from build123d import *

# Parameters (mm, degrees)
SKETCH1_R                                   = 155.575
SKETCH1_R_2                                 = 7.9375
BOSS_EXTRUDE1_DEPTH                         = 4.7625
FILLET1_R                                   = 12.7
FILLET4_R                                   = 2.54
CSK_FOR_1_4_FLAT_HEAD_MACHINE_SCREW_2_COUNT = 2
CSK_FOR_1_4_FLAT_HEAD_MACHINE_SCREW_2_PITCH = 255.715651102
CSK_FOR_1_4_FLAT_HEAD_MACHINE_SCREW_3_COUNT = 2
CSK_FOR_1_4_FLAT_HEAD_MACHINE_SCREW_3_PITCH = 255.715651102


with BuildPart() as part:
    # Sketch1 → Boss-Extrude1 (new body)
    with BuildSketch(Plane.XY):
        Circle(SKETCH1_R)
        with BuildLine():
            ThreePointArc((-125.107792883, -62.16212802), (-120.983748909, 69.85), (-8.719914422, 139.427590858))
            Line((-8.719914422, 139.427590858), (-12.49892387, 7.216257061))
            Line((-12.49892387, 7.216257061), (-125.107792883, -62.16212802))
        make_face(mode=Mode.SUBTRACT)
        with BuildLine():
            ThreePointArc((8.719914422, 139.427590858), (120.983748909, 69.85), (125.107792883, -62.16212802))
            Line((125.107792883, -62.16212802), (12.49892387, 7.216257061))
            Line((12.49892387, 7.216257061), (8.719914422, 139.427590858))
        make_face(mode=Mode.SUBTRACT)
        with BuildLine():
            ThreePointArc((116.38787846, -77.265462838), (0, -139.7), (-116.38787846, -77.265462838))
            Line((-116.38787846, -77.265462838), (0, -14.432514122))
            Line((0, -14.432514122), (116.38787846, -77.265462838))
        make_face(mode=Mode.SUBTRACT)
        with BuildLine():
            Line((-12.585726429, 4.179407795), (-12.694815268, 0.362857143))
            ThreePointArc((-12.694815268, 0.362857143), (-10.998522628, -6.35), (-6.03316413, -11.17546109))
            Line((-6.03316413, -11.17546109), (-2.673389891, -12.98926271))
            Line((-2.673389891, -12.98926271), (-112.467905529, -72.262730545))
            ThreePointArc((-112.467905529, -72.262730545), (-120.983748909, -69.85), (-118.815313164, -61.268698026))
            Line((-118.815313164, -61.268698026), (-12.585726429, 4.179407795))
        make_face(mode=Mode.SUBTRACT)
        with BuildLine():
            ThreePointArc((118.815313164, -61.268698026), (120.983748909, -69.85), (112.467905529, -72.262730545))
            Line((112.467905529, -72.262730545), (2.673389891, -12.98926271))
            Line((2.673389891, -12.98926271), (6.03316413, -11.17546109))
            ThreePointArc((6.03316413, -11.17546109), (10.998522628, -6.35), (12.694815268, 0.362857143))
            Line((12.694815268, 0.362857143), (12.585726429, 4.179407795))
            Line((12.585726429, 4.179407795), (118.815313164, -61.268698026))
        make_face(mode=Mode.SUBTRACT)
        Circle(SKETCH1_R_2, mode=Mode.SUBTRACT)
        with BuildLine():
            ThreePointArc((-6.347407634, 133.531428571), (0, 139.7), (6.347407634, 133.531428571))
            Line((6.347407634, 133.531428571), (9.938137929, 7.907174875))
            ThreePointArc((9.938137929, 7.907174875), (0, 12.7), (-9.938137929, 7.907174875))
            Line((-9.938137929, 7.907174875), (-6.347407634, 133.531428571))
        make_face(mode=Mode.SUBTRACT)
    extrude(amount=-BOSS_EXTRUDE1_DEPTH)

    # Fillet1
    fillet1_edges = [part.edges().sort_by_distance(p)[0] for p in [
        (12.49892387, 7.216257061, -2.38125),
        (0, -14.432514122, -2.38125),
        (-12.49892387, 7.216257061, -2.38125),
    ]]
    fillet(fillet1_edges, radius=FILLET1_R)

    # Fillet4
    fillet4_edges = [part.edges().sort_by_distance(p)[0] for p in [
        (12.585726429, 4.179407795, -2.38125),
        (2.673389891, -12.98926271, -2.38125),
        (-2.673389891, -12.98926271, -2.38125),
        (-12.585726429, 4.179407795, -2.38125),
        (-9.938137929, 7.907174875, -2.38125),
        (9.938137929, 7.907174875, -2.38125),
    ]]
    fillet(fillet4_edges, radius=FILLET4_R)

    # Sketch4 → CSK for 1/4 Flat Head Machine Screw (100)1 (revolve, cut)
    with BuildSketch(Plane(origin=(0, 147.6375, 0), x_dir=(0, -1, 0), z_dir=(1, 0, 0))):
        Polygon((0, 0), (0, 4.7625), (3.3782, 4.7625), (3.3782, 2.568232241), (6.4389, 0), align=None)
    csk_for_1_4_flat_head_machine_screw_100 = revolve(axis=Axis((0, 147.6375, 6.35), (0, 0, -1)), mode=Mode.SUBTRACT)

    # CSK for 1_4 Flat Head Machine Screw  2: CSK for 1/4 Flat Head Machine Screw (100)1 ×2
    with Locations(*[Vector(0.5, -0.866025404, 0) * (i * CSK_FOR_1_4_FLAT_HEAD_MACHINE_SCREW_2_PITCH) for i in range(1, CSK_FOR_1_4_FLAT_HEAD_MACHINE_SCREW_2_COUNT)]):
        add(csk_for_1_4_flat_head_machine_screw_100, mode=Mode.SUBTRACT)

    # CSK for 1_4 Flat Head Machine Screw  3: CSK for 1/4 Flat Head Machine Screw (100)1 ×2
    with Locations(*[Vector(-0.5, -0.866025404, 0) * (i * CSK_FOR_1_4_FLAT_HEAD_MACHINE_SCREW_3_PITCH) for i in range(1, CSK_FOR_1_4_FLAT_HEAD_MACHINE_SCREW_3_COUNT)]):
        add(csk_for_1_4_flat_head_machine_screw_100, mode=Mode.SUBTRACT)


solid = part.part
The listing builds one solid part. Answer for the finished solid, in the listing's coordinates (mm). A direction names the side the tool comes from. Give positions to 0.01 mm unless a question says otherwise; leave off trailing zeros. Write each loop counter-clockwise with the first axis right and the second up, starting at its lowest first coordinate (ties: lowest second). Pieces come first, ordered by that corner, then holes.
1) Section A-A (x = -57.5) is taken. Write down the section's boundary in (y, z), and give its area (3 significant figures).
2) For a pull along Y with two mould halves and no side action, classify faces 3 (the face through (-130.3, -71.2, -2.4)), 4 (the face through (-1, -11, 0)), 5 (the face through (72.47, -29.73, -2.35)) as pulls with the +Y half, pulls with the -Y half, needs draft (parallel to the pull), parting line crosses it, or undercut.
3) Section B-B (y = -52) is taken. Write down the section's boundary in (x, z).
4) Section C-C (y = 111) is taken. Write down the section's boundary in (x, z).
5) Section D-D (y = -113) is taken. Write down the section's boundary in (x, z).
6) A tool of negligible diameter and unlimited length cuts with its end or side. For faces 1 (the face through (60.44, -47.06, -2.35)), 2 (the face through (-1, -11, -4.762)), from which of +Z, -Z, +X, -X, +Y, -Y can it reach the whole face along a straight path? Write none if from no direction.
7) Given P1, Ø1.5, axis at x = -100, z = -2, coming from the +Y side; P2, Ø5.5, axis at x = -127.86, y = -73.82, coming from the -Z side; P3, Ø8, axis at x = 127.86, y = -73.82, coming from the +Z side, each flat-ended and moving along its own axis, determine where each tip first touches the part or whether it passes through.
8) Find the intervals of material crossed by L1, parallel to Y at x = 113.5, z = -2.2; L2, parallel to Y at x = -69.5, z = -3.9; L3, parallel to Y at x = 124.5, z = -0.9, in increasing order.
Response:
1. outline: (-144.56, -4.76) - (-127.32, -4.76) - (-127.32, 0) - (-144.56, 0) - close; (-45.47, -4.76) - (-42.59, -4.76) - (-42.59, 0) - (-45.47, 0) - close; (-23.49, -4.76) - (-20.51, -4.76) - (-20.51, 0) - (-23.49, 0) - close; (127.32, -4.76) - (144.56, -4.76) - (144.56, 0) - (127.32, 0) - close
1. area: 192 mm2
2. face 3: undercut
2. face 4: needs draft
2. face 5: undercut
3. outline: (-146.63, -4.76) - (-129.66, -4.76) - (-129.66, 0) - (-146.63, 0) - close; (-108.61, -4.76) - (-103.77, -4.76) - (-103.77, 0) - (-108.61, 0) - close; (-74.93, -4.76) - (-69.59, -4.76) - (-69.59, 0) - (-74.93, 0) - close; (69.59, -4.76) - (74.93, -4.76) - (74.93, 0) - (69.59, 0) - close; (103.77, -4.76) - (108.61, -4.76) - (108.61, 0) - (103.77, 0) - close; (129.66, -4.76) - (146.63, -4.76) - (146.63, 0) - (129.66, 0) - close
4. outline: (-109.01, -4.76) - (-84.82, -4.76) - (-84.82, 0) - (-109.01, 0) - close; (-9.53, -4.76) - (-6.99, -4.76) - (-6.99, 0) - (-9.53, 0) - close; (6.99, -4.76) - (9.53, -4.76) - (9.53, 0) - (6.99, 0) - close; (84.82, -4.76) - (109.01, -4.76) - (109.01, 0) - (84.82, 0) - close
5. outline: (-106.93, -4.76) - (-82.14, -4.76) - (-82.14, 0) - (-106.93, 0) - close; (82.14, -4.76) - (106.93, -4.76) - (106.93, 0) - (82.14, 0) - close
6. face 1: +Z, -Z
6. face 2: -Z, +X, -X, +Y, -Y
7. P1: stops at y = 119.8
7. P2: passes through
7. P3: stops at z = -2.04
8. L1: y = -106.4 to -81.45, -75.71 to -72.71, -57.99 to -55.01, 81.45 to 106.4
8. L2: y = -139.19 to -121.19, -51.95 to -49.07, -30.89 to -27.9, 121.19 to 139.19
8. L3: y = -93.29 to -78, -69.63 to -61.79, 63.37 to 93.29
